For this review, take the finished solid that the model builds, in its own axes (mm). Give positions to 0.01 mm unless a question says otherwise; leave off trailing zeros. Loops run counter-clockwise (first coordinate to the right, second up) from the corner with the lowest first, then second, coordinate; pieces in that order, holes last. Notation, with made-up numbers: (71, 56) - (103, 56) arc R30 cw to (103, 87) - close; hole circle Ø3 at (56, 44). An arc over 180 degrees is marked (long way). Answer in a Markdown table with one row per item.
```python
from build123d import *

# Parameters (mm, degrees)
SKETCH2_R                = 1.27
BOSS_EXTRUDE1_DEPTH      = 1.5875
BOSS_EXTRUDE1_DEPTH_BACK = 5.55625


with BuildPart() as part:
    # Sketch1 → Revolve1 (revolve)
    with BuildSketch(Plane(origin=(0, 0, 0), x_dir=(1, 0, 0), z_dir=(0, 1, 0))):
        Polygon((0, 0), (3.96875, 0), (3.96875, 15.08125), (1.984375, 14.148388583), (0, 15.08125), align=None)
    revolve(axis=Axis((0, 0, 0), (1, 0, 0)))

    # Sketch2 → Boss-Extrude1 (add, two sides)
    with BuildSketch(Plane(origin=(3.96875, 0, 0), x_dir=(0, 0, -1), z_dir=(1, 0, 0))) as boss_extrude1_sk:
        Circle(SKETCH2_R)
    extrude(amount=BOSS_EXTRUDE1_DEPTH)
    extrude(boss_extrude1_sk.sketch, amount=-BOSS_EXTRUDE1_DEPTH_BACK)


solid = part.part
```
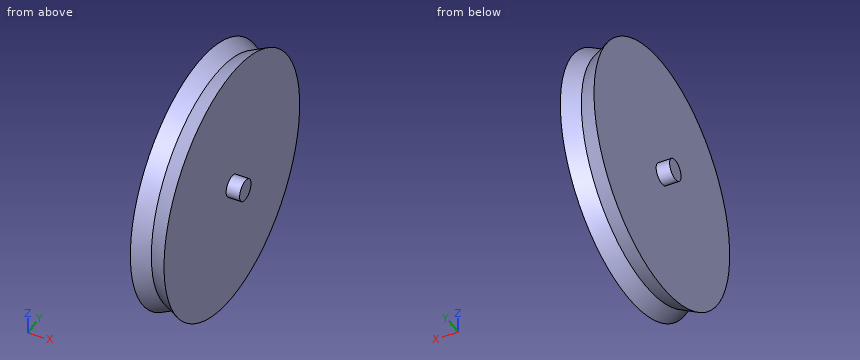
1. We need section C-C, the plane x = -0.5. Give the boundary of the cut face in (y, z), and give its area (3 significant figures).
Values:
| item | result |
|---|---|
| outline | circle Ø2.54 at (0, 0) |
| area | 5.07 mm^2 |
2. We need section A-A, the plane z = 0. Give the boundary of the cut face in (x, y).
Values:
| item | result |
|---|---|
| outline | (-1.59, -1.27) - (0, -1.27) - (0, -15.08) - (1.98, -14.15) - (3.97, -15.08) - (3.97, -1.27) - (5.56, -1.27) - (5.56, 1.27) - (3.97, 1.27) - (3.97, 15.08) - (1.98, 14.15) - (0, 15.08) - (0, 1.27) - (-1.59, 1.27) - close |
3. Clearance check with flat-ended pins moving along their axes: pin 1 (6 mm diameter, centred on y = -8.5, z = -6, fed in from +X); pin 2 (2 mm diameter, centred on x = 5, y = 0, fed in from +Z); pin 3 (9 mm diameter, centred on y = 4, z = 6.5, fed in from -X); pin 4 (5 mm diameter, centred on y = 0.5, z = -2.5, fed in from -X). State where each tip first meets the part, or that it passes through.
Values:
| item | result |
|---|---|
| pin 1 | stops at x = 3.97 |
| pin 2 | stops at z = 1.27 |
| pin 3 | stops at x = 0 |
| pin 4 | stops at x = -1.59 |
4. Wall thickness on line 1 (X direction, y = 11.5, z = 3.5); line 2 (Z direction, x = 3, y = 2.5); line 3 (Y direction, x = 2.5, z = 7): over which ranges is each line inside the solid? List them lowest first. Write a range as [from, to].
Values:
| item | result |
|---|---|
| line 1 | x = [0, 3.97] |
| line 2 | z = [-14.41, 14.41] |
| line 3 | y = [-12.57, 12.57] |
